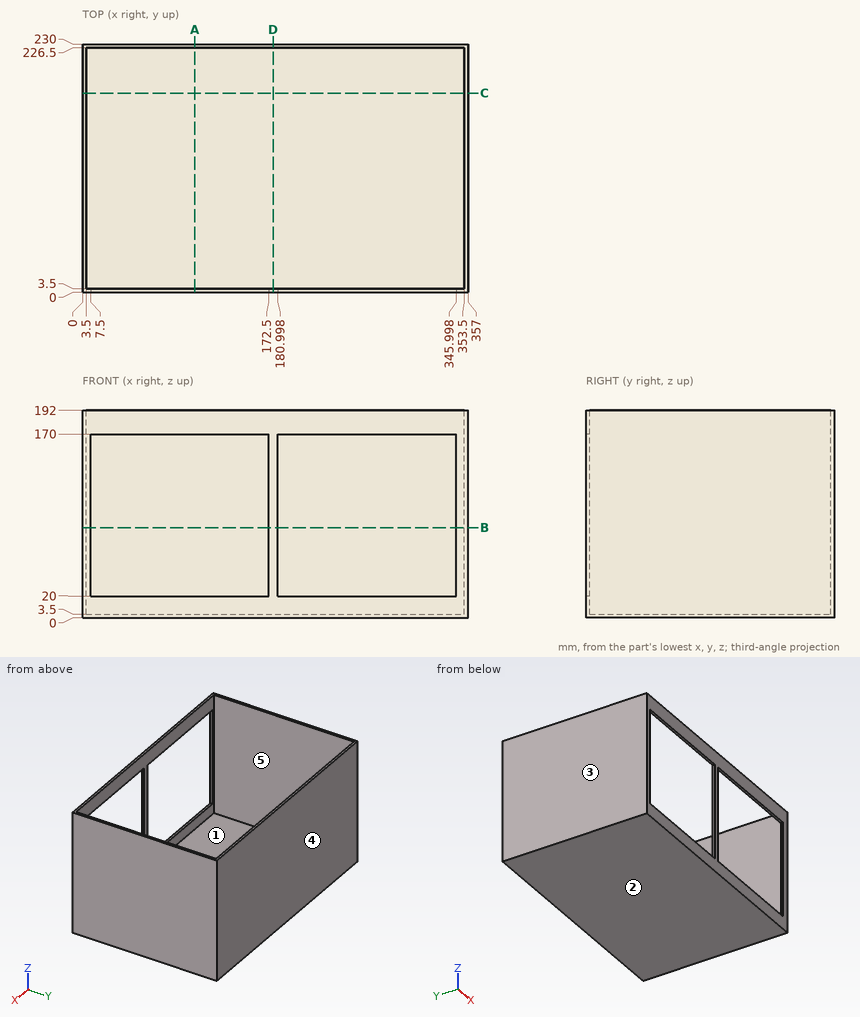
Source: three-view drawing plus pictorial views. Frame: mm from the lowest corner of the part. A direction names the side the tool comes from. Round coordinates to 2 decimals unless told otherwise and drop trailing zeros. Loops run counter-clockwise (first coordinate to the right, second up) from the corner with the lowest first, then second, coordinate; pieces in that order, holes last. Notation, with made-up numbers: (-16, 31) - (40, 31) arc R35 cw to (40, 64) - close; hole circle Ø6 at (55.5, -4.5). An arc over 180 degrees is marked (long way). Write item = value, one per line. Start each with the question number.
Item 1: Section query D-D on x = 176.5. Output: boundary loops of the cut face in (y, z).
Item 2: Reachability of the marked faces 4 and 5 from +Z, -Z, +X, -X, +Y, -Y: full face, straight path, thin tool, end or side. Return the list, or none.
Item 3: First-contact query: pin 1 Ø2 at (x, z) = (148.5, 61.5) entering from -Y. Flat tip, straight axial feed; report the tip coordinate or a pass-through.
Item 4: Section query B-B on z = 83.5. Output: boundary loops of the cut face in (x, y).
Item 5: Material intervals for line 1 (X direction, y = 203, z = 95); line 2 (Y direction, x = 37.5, z = 19); line 3 (Z direction, x = 303.5, y = 101), sorted ascending.
Item 6: Mould query, pull axis X, two halves, no side actions, for the marked faces 1, 2 and 3. Classes: released by +X, released by -X, zero draft, split by the parting line, or undercut.
Item 7: Section query C-C on y = 184.5. Output: boundary loops of the cut face in (x, z).
Item 8: Section query A-A on x = 104. Output: boundary loops of the cut face in (y, z), plus the area to 3 significant figures.
Results list:
q1.outline = (0, 0) - (230, 0) - (230, 192) - (226.5, 192) - (226.5, 3.5) - (3.5, 3.5) - (3.5, 192) - (0, 192) - close
q2.face_4 = +Z, -Z, +X, -X, +Y
q2.face_5 = +Z
q3.pin_1 = 226.5
q4.outline = (0, 0) - (7.5, 0) - (7.5, 3.5) - (3.5, 3.5) - (3.5, 226.5) - (353.5, 226.5) - (353.5, 3.5) - (346, 3.5) - (346, 0) - (357, 0) - (357, 230) - (0, 230) - close; (172.5, 0) - (181, 0) - (181, 3.5) - (172.5, 3.5) - close
q5.line_1 = 0 to 3.5, 353.5 to 357
q5.line_2 = 0 to 3.5, 226.5 to 230
q5.line_3 = 0 to 3.5
q6.face_1 = undercut
q6.face_2 = zero draft
q6.face_3 = released by -X
q7.outline = (0, 0) - (357, 0) - (357, 192) - (353.5, 192) - (353.5, 3.5) - (3.5, 3.5) - (3.5, 192) - (0, 192) - close
q8.outline = (0, 0) - (230, 0) - (230, 192) - (226.5, 192) - (226.5, 3.5) - (3.5, 3.5) - (3.5, 20) - (0, 20) - close; (0, 170) - (3.5, 170) - (3.5, 192) - (0, 192) - close
q8.area = 1,600 mm²
